Autodesk Inventor part; units mm, degrees
ref_plane "YZ Plane" through (0, 0, 0) normal (1, 0, 0) x (0, 1, 0)
ref_plane "XZ Plane" through (0, 0, 0) normal (0, 1, 0) x (-1, 0, 0)
ref_plane "XY Plane" through (0, 0, 0) normal (0, 0, 1) x (1, 0, 0)
sketch "Sketch1" plane through (0, 0, 0) normal (0, 0, 1) x (1, 0, 0)
  line L0 (0, 0) -> (50.8, 0)
  line L1 (50.8, 0) -> (50.8, 152.4)
  line L2 (50.8, 203.2) -> (0, 203.2)
  line L3 (0, 203.2) -> (0, 0)
  line L4 (0, 203.2) -> (355.6, 203.2)
  line L5 (355.6, 203.2) -> (355.6, 152.4)
  line L6 (355.6, 152.4) -> (50.8, 152.4)
  line L7 (0, 152.4) -> (0, 203.2)
  dimension "d0" = 50.8
  dimension "d1" = 203.2
  dimension "d2" = 355.6
  dimension "d3" = 50.8
extrude "Extrusion1" add sketch "Sketch1" along normal blind 3.175
sketch "Sketch2" plane through (0, 0, 3.175) normal (0, 0, 1) x (1, 0, 0)
  line L0 (355.6, 203.2) -> (0, 203.2)
  line L1 (0, 203.2) -> (0, 0)
  point P0 (25.4, 165.1)
  dimension "d20" = 38.1
  dimension "d21" = 25.4
hole "Hole1" at (25.4, 165.1, 3.175) direction (0, 0, -1) diameter 28.575 end through all
sketch "Sketch3" plane through (0, 0, 3.175) normal (0, 0, 1) x (1, 0, 0)
  line L0 (50.8, 0) -> (50.8, 152.4)
  line L1 (0, 0) -> (50.8, 0)
  point P0 (25.4, 25.4)
  dimension "d22" = 25.4
  dimension "d23" = 25.4
hole "Hole2" at (25.4, 25.4, 3.175) direction (0, 0, -1) diameter 28.575 end through all
fillet "Fillet1" radius 6.35 5 edges at (355.6, 152.4, 1.5875) (355.6, 203.2, 1.5875) (50.8, 0, 1.5875) (0, 0, 1.5875) (0, 203.2, 1.5875)
sketch "Sketch4" plane through (0, 0, 3.175) normal (0, 0, 1) x (1, 0, 0)
  line L0 (349.25, 203.2) -> (6.35, 203.2)
  line L1 (355.6, 158.75) -> (355.6, 196.85)
  point P0 (0, 0)
  point P1 (330.2, 177.8)
  dimension "d32" = 25.4
  dimension "d33" = 25.4
hole "Hole3" at (330.2, 177.8, 3.175) direction (0, 0, -1) diameter 28.575 end through all
properties part number "Arm"
CAD build for the part. Positions are in the model's coordinates, mm. Coordinates: 2 decimals unless noted, no trailing zeros. Write each loop counter-clockwise with the first axis right and the second up, starting at its lowest first coordinate (ties: lowest second). Pieces come first, ordered by that corner, then holes.
(1) Cut at B-B, the plane x = 25.4. List the corners of the cut face in (y, z) (1 decimal), and give its area (3 significant figures).
(2) Two-plate mould, pull along Y, no slides. Class faces 1 (the face through (137, 155, 3.175)), 2 (the face through (11.234, 27.26, 1.565)), 3 (the face through (1.91, 201.39, 1.61)): +Y half, -Y half, draft (parallel to the pull), parting line (faces both ways), or undercut.
(3) Cut at D-D, the plane x = 330.2. List the corners of the cut face in (y, z) (1 decimal), and give its area (3 significant figures).
(4) Cut at A-A, the plane z = 2.45. Count the separate pieces of the cut face and the enclosed holes in it, and give its area (3 significant figures).
(5) Drill centre lines: probe 1 along Y at (x, z) = (25.4, 1.25); probe 2 along X at (y, z) = (165.1, 0.7); probe 3 along X at (y, z) = (25.4, 1.9). Where is each one in solid material? Low to high.
(6) Cut at C-C, the plane y = 25.4. List the corners of the cut face in (x, z) (1 decimal).
(7) Flat gauge pin, fed straight in: pin 1 (1 mm diameter, centred on x = 66.5, z = 1.5, fed in from -Y). Where does the tip first touch, or does it go through?
Geometry says:
1. outline: (0, 0) - (11.1, 0) - (11.1, 3.2) - (0, 3.2) - close; (39.7, 0) - (150.8, 0) - (150.8, 3.2) - (39.7, 3.2) - close; (179.4, 0) - (203.2, 0) - (203.2, 3.2) - (179.4, 3.2) - close
1. area: 464 mm2
2. face 1: draft
2. face 2: undercut
2. face 3: +Y half
3. outline: (152.4, 0) - (163.5, 0) - (163.5, 3.2) - (152.4, 3.2) - close; (192.1, 0) - (203.2, 0) - (203.2, 3.2) - (192.1, 3.2) - close
3. area: 70.6 mm2
4. separate pieces: 1
4. enclosed holes: 3
4. area: 23,800 mm2
5. probe 1: y = 0 to 11.11, 39.69 to 150.81, 179.39 to 203.2
5. probe 2: x = 0 to 11.11, 39.69 to 323.65, 336.75 to 355.6
5. probe 3: x = 0 to 11.11, 39.69 to 50.8
6. outline: (0, 0) - (11.1, 0) - (11.1, 3.2) - (0, 3.2) - close; (39.7, 0) - (50.8, 0) - (50.8, 3.2) - (39.7, 3.2) - close
7. pin 1: stops at y = 152.4
